Can you work these out from the model? Positions are in its coordinate system, mm. A direction names the side the tool comes from. Round coordinates to 2 decimals unless told otherwise and drop trailing zeros. Loops run counter-clockwise (first coordinate to the right, second up) from the corner with the lowest first, then second, coordinate; pieces in that order, holes last.
(1) I want a section at D-D on x = 26. Write out the boundary of the cut face in (y, z), plus the area to 4 significant figures.
(2) Which directions (+Z, -Z, +X, -X, +Y, -Y) give clear straight access to the entire face, cutting with the end or side of a thin tool? Please do faces 5 (the face through (20, 1, 100)), 6 (the face through (19.8, -14.5, 3)), 7 (the face through (20.1, 1.5, 87.5)).
(3) Thinking about a two-plate mould opening in Z: for faces 1 (the face through (17.5, 1, 50)), 2 (the face through (3, -9, 10)), 3 (the face through (1.48, -14.79, 16.69)), 4 (the face through (22.5, 1, 50)), which applies, released by +Z, released by -Z, zero draft, split by the parting line, or undercut?
(4) I want a section at B-B on z = 40. Write out the boundary of the cut face in (x, y), plus the area to 3 significant figures.
(5) Will these pins go through, and if not, where does the flat tip stop? pin 1 Ø3 at (x, y) = (20, -16.5) entering from +Z; pin 2 Ø3 at (x, z) = (21.5, 71.5) entering from -Y; pin 3 Ø6 at (x, y) = (29, -3.5) entering from +Z; pin 4 Ø8 at (x, y) = (10, -20.5) entering from +Z.
(6) I want a section at C-C on y = -13.5. Write out the boundary of the cut face in (x, z), plus the area to 3 significant figures.
(7) If I drill on line 1 along X through (y, z) = (-16.5, 12.5); line 2 along Y through (x, z) = (20, 1.45); line 3 along Y through (x, z) = (26, 8), over which ranges is the centre line in solid material (lowest first)?
(8) I want a section at A-A on x = 20. Write out the boundary of the cut face in (y, z), plus the area to 3 significant figures.
from build123d import *

# Parameters (mm, degrees)
SKETCH1_W               = 40
SKETCH1_H               = 100
BOSS_EXTRUDE1_DEPTH     = 3
SKETCH2_W               = 40
SKETCH2_H               = 3
BOSS_EXTRUDE2_DEPTH     = 30
CHAMFER1_SIZE           = 5
SKETCH3_W               = 3
SKETCH3_H               = 33
BOSS_EXTRUDE3_DEPTH     = 30
CUT_EXTRUDE1_DEPTH      = 50
CUT_EXTRUDE1_DEPTH_BACK = 30
SKETCH5_R               = 1.75
CUT_EXTRUDE2_DEPTH      = 30


with BuildPart() as part:
    # Sketch1 → Boss-Extrude1 (new body)
    with BuildSketch(Plane(origin=(0, 0, 0), x_dir=(1, 0, 0), z_dir=(0, 1, 0))):
        with Locations((20, -50)):
            Rectangle(SKETCH1_W, SKETCH1_H)
        with BuildLine():
            Line((17.5, -85), (17.5, -15))
            ThreePointArc((17.5, -15), (20, -12.5), (22.5, -15))
            Line((22.5, -15), (22.5, -85))
            ThreePointArc((22.5, -85), (20, -87.5), (17.5, -85))
        make_face(mode=Mode.SUBTRACT)
    extrude(amount=BOSS_EXTRUDE1_DEPTH)

    # Sketch2 → Boss-Extrude2 (add)
    with BuildSketch(Plane.XZ):
        with Locations((20, 1.5)):
            Rectangle(SKETCH2_W, SKETCH2_H)
    extrude(amount=BOSS_EXTRUDE2_DEPTH)

    # Chamfer1
    chamfer1_edges = [part.edges().sort_by_distance(p)[0] for p in [
        (20, 0, 3),
    ]]
    chamfer(chamfer1_edges, length=CHAMFER1_SIZE)

    # Sketch3 → Boss-Extrude3 (add)
    with BuildSketch(Plane(origin=(0, 0, 0), x_dir=(-1, 0, 0), z_dir=(0, 0, -1))):
        with Locations((-1.5, -13.5)):
            Rectangle(SKETCH3_W, SKETCH3_H)
        with Locations((-38.5, -13.5)):
            Rectangle(SKETCH3_W, SKETCH3_H)
    extrude(amount=-BOSS_EXTRUDE3_DEPTH)

    # Sketch4 → Cut-Extrude1 (cut, two sides: drawn at the far end of the back side and taken through both)
    with BuildSketch(Plane(origin=(3, 0, 0), x_dir=(0, 0, -1), z_dir=(1, 0, 0)).offset(-CUT_EXTRUDE1_DEPTH_BACK)):
        Polygon((-30, 0), (-3, -30), (-30, -30), align=None)
    extrude(amount=CUT_EXTRUDE1_DEPTH + CUT_EXTRUDE1_DEPTH_BACK, mode=Mode.SUBTRACT)

    # Sketch5 → Cut-Extrude2 (cut)
    with BuildSketch(Plane.XY.offset(3)):
        with Locations((20, -16.495296504)):
            Circle(SKETCH5_R)
    extrude(amount=-CUT_EXTRUDE2_DEPTH, mode=Mode.SUBTRACT)


solid = part.part
Filled sheet:
1. outline: (-30, 0) - (3, 0) - (3, 100) - (0, 100) - (0, 8) - (-5, 3) - (-30, 3) - close
1. area: 402.5 mm2
2. face 5: +Z, +X, -X, +Y, -Y
2. face 6: +Z, -Y
2. face 7: +Y, -Y
3. face 1: undercut
3. face 2: zero draft
3. face 3: released by +Z
3. face 4: undercut
4. outline: (0, 0) - (17.5, 0) - (17.5, 3) - (0, 3) - close; (22.5, 0) - (40, 0) - (40, 3) - (22.5, 3) - close
4. area: 105 mm2
5. pin 1: passes through
5. pin 2: stops at y = 0
5. pin 3: stops at z = 7.5
5. pin 4: stops at z = 3
6. outline: (0, 0) - (40, 0) - (40, 17.85) - (37, 17.85) - (37, 3) - (3, 3) - (3, 17.85) - (0, 17.85) - close
6. area: 209 mm2
7. line 1: x = 0 to 3, 37 to 40
7. line 2: y = -30 to -18.25, -14.75 to 3
7. line 3: y = 0 to 3
8. outline: (-30, 0) - (-18.25, 0) - (-18.25, 3) - (-30, 3) - close; (-14.75, 0) - (3, 0) - (3, 12.5) - (0, 12.5) - (0, 8) - (-5, 3) - (-14.75, 3) - close; (0, 87.5) - (3, 87.5) - (3, 100) - (0, 100) - close
8. area: 167 mm2
